Could you check a few things on this model? Use its own coordinates, in mm. Give positions to 0.01 mm unless a question says otherwise; leave off trailing zeros. Write each loop counter-clockwise with the first axis right and the second up, starting at its lowest first coordinate (ties: lowest second). Pieces come first, ordered by that corner, then holes. Notation, with made-up numbers: (59.25, 56.5) - (115.25, 56.5) arc R35 ccw to (115.25, 94.5) - close; hole circle Ø8 at (-4, -23.5). An arc over 180 degrees is marked (long way). Answer in a Markdown table with one row per item.
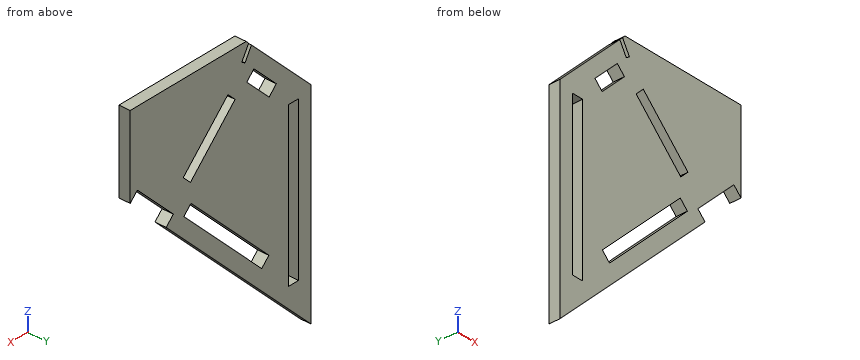
from build123d import *

# Parameters (mm, degrees)
SKETCH1_W           = 8
SKETCH1_H           = 113.93
BOSS_EXTRUDE1_DEPTH = 8


with BuildPart() as part:
    # Sketch1 → Boss-Extrude1 (new body)
    with BuildSketch(Plane(origin=(0, 0, 0), x_dir=(1, 0, 0), z_dir=(0, 1, 0))):
        Polygon((-91.75, 0), (0, 0), (0, 58.25), (-0.001499297, 58.251499297), (-5.658353547, 52.594645048), (-34.126472557, 81.062764058), (-28.469618308, 86.719618308), (-143.078881246, 201.328881246), (-143.078881246, 51.328881246), (-95.946152423, 4.196152423), (-90.846474596, 13.02905352), (-88.248398385, 11.52905352), (-93.75, 2), align=None)
        Polygon((-97.917542408, 20.100121332), (-115.595211938, 37.777790862), (-109.938357688, 43.434645111), (-92.260688159, 25.756975582), align=None, mode=Mode.SUBTRACT)
        Polygon((-77.337199542, 26.538328575), (-82.994053791, 32.195182824), (-47.638714732, 67.550521884), (-41.981860482, 61.893667634), align=None, mode=Mode.SUBTRACT)
        with Locations((-129.272881467, 112.420460392)):
            Rectangle(SKETCH1_W, SKETCH1_H, mode=Mode.SUBTRACT)
        Polygon((-48.085105233, 80.883975658), (-109.716532281, 142.515402707), (-104.059678032, 148.172256956), (-42.428250984, 86.540829908), align=None, mode=Mode.SUBTRACT)
    extrude(amount=BOSS_EXTRUDE1_DEPTH)


solid = part.part
1) Imagine slicing it at D-D (x = -40). List the corners of the cut face in (y, z) for me.
Check values:
| item | result |
|---|---|
| outline | (0, -98.25) - (8, -98.25) - (8, 0) - (0, 0) - close |
2) Imagine slicing it at C-C (y = 1.5). State how many separate pieces and enclosed holes the cut face has, then the cut area to 3 significant figures.
Check values:
| item | result |
|---|---|
| separate pieces | 1 |
| enclosed holes | 4 |
| area | 14,700 mm2 |
3) Imagine slicing it at A-A (x = -58.5). List the corners of the cut face in (y, z) for me, then the cut area to 3 significant figures.
Check values:
| item | result |
|---|---|
| outline | (0, -116.75) - (8, -116.75) - (8, -102.61) - (0, -102.61) - close; (0, -91.3) - (8, -91.3) - (8, -56.69) - (0, -56.69) - close; (0, -45.38) - (8, -45.38) - (8, 0) - (0, 0) - close |
| area | 753 mm2 |
4) Imagine slicing it at B-B (z = -95). List the corners of the cut face in (x, y) for me.
Check values:
| item | result |
|---|---|
| outline | (-143.08, 0) - (-133.27, 0) - (-133.27, 8) - (-143.08, 8) - close; (-125.27, 0) - (-62.2, 0) - (-62.2, 8) - (-125.27, 8) - close; (-50.89, 0) - (-36.75, 0) - (-36.75, 8) - (-50.89, 8) - close |
5) If I drill on line 1 (X direction, y = 3.75, z = -119); line 2 (X direction, y = 1.75, z = -31.5); line 3 (Z direction, x = -101.5, y = 6), over which ranges is the centre line in solid material (lowest first)?
Check values:
| item | result |
|---|---|
| line 1 | x = -143.08 to -133.27, -125.27 to -86.2, -74.89 to -60.75 |
| line 2 | x = -123.25 to -109.32, -98 to -82.3, -72.38 to 0 |
| line 3 | z = -159.75 to -145.61, -134.3 to -35, -23.68 to -9.75 |
6) Will these pins go through, and if not, where does the flat tip stop? P1, Ø4, axis at x = -127.5, y = 6, coming from the -Z side; P2, Ø1.5, axis at x = -56.5, y = 4, coming from the -Z side; P3, Ø1.5, axis at y = 4, z = -108.5, coming from the +X side.
Check values:
| item | result |
|---|---|
| P1 | stops at z = -187.75 |
| P2 | stops at z = -115.5 |
| P3 | stops at x = -49.5 |
